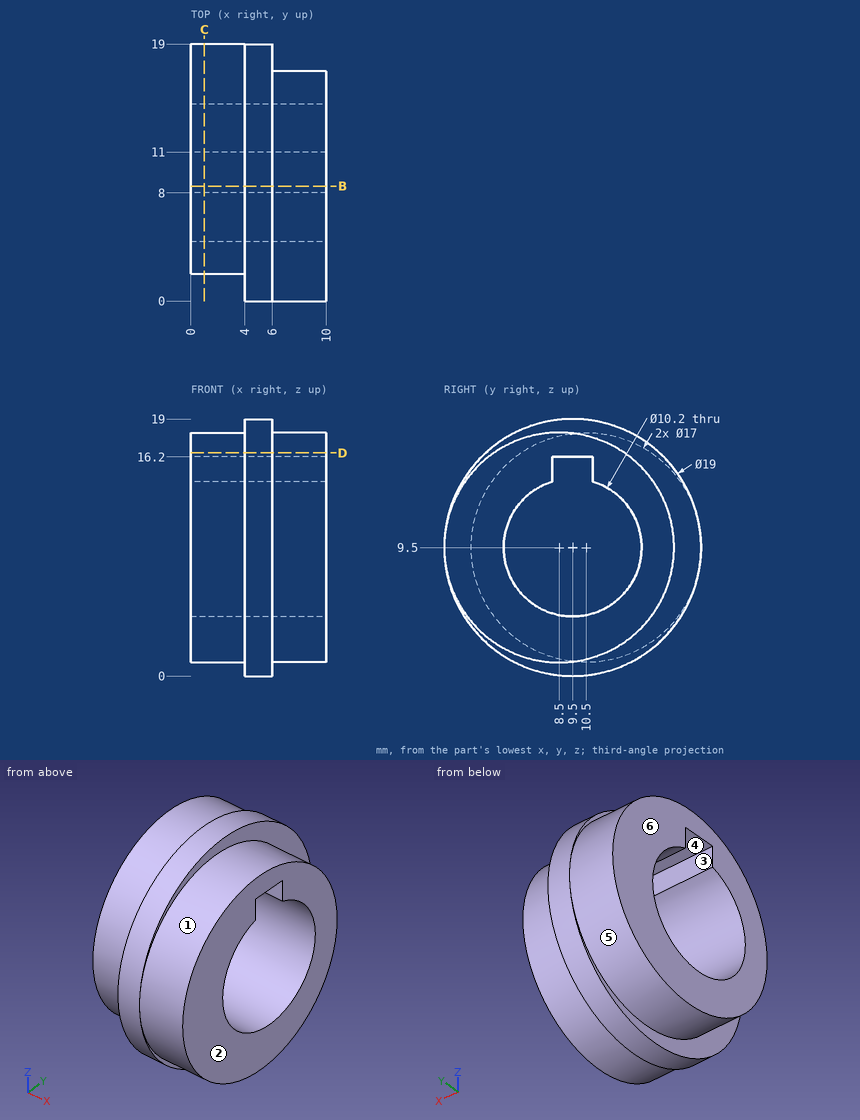
Geometry check sheet. Reference: drawing and pictorial views, mm from the part's lowest x, y, z. A direction names the side the tool comes from. Give positions to 0.01 mm unless a question says otherwise; leave off trailing zeros. Order: outer loops, then holes, each group sorted by start corner. A loop starts at its lowest first (then second) coordinate and runs counter-clockwise, first axis right, second up. Notation, with made-up numbers: M -4.5,69 L 21.5,69 A31 cw 21.5,108 Z; hole C -3,-32.75 d9. An arc over 180 degrees is marked long. Answer in a Markdown table with one row per item. Add a question column.
Q1. Sectioned sample at B-B, the plane y = 8.5. Record the boundary of the cut face in (x, z).
Q2. Access from +Z, -Z, +X, -X, +Y, -Y to the whole of each face (thin tool, end or side, straight path). Record for the marked faces 4, 5 and 6.
Q3. Sectioned sample at D-D, the plane z = 16.5. Record the boundary of the cut face in (x, y), and give its area (3 significant figures).
Q4. Thickness scan on L1, parallel to Z at x = 5, y = 9.5; L2, parallel to Y at x = 3.25, z = 9.5; L3, parallel to Z at x = 7.75, y = 7.25. Record the ranges inside material, lowest first.
Q5. Gauge pin test, flat ends, axial feed: pin 1 Ø1.5 at (x, y) = (8.5, 10) entering from -Z; pin 2 Ø6 at (y, z) = (16.5, 16.5) entering from -X; pin 3 Ø0.9 at (x, z) = (4, 15.5) entering from +Y; pin 4 Ø4 at (x, z) = (3, 17) entering from -Y. Record the tip position at first contact, or that the pin passes through.
Q6. Release check for a two-part mould opening along Z. For the marked faces 1, 2 and 3 record: released by +Z, released by -Z, zero draft, split by the parting line, or undercut.
Q7. Sectioned sample at C-C, the plane x = 1. Record the boundary of the cut face in (y, z), and give its area (3 significant figures).
Verdict:
| question | item | result |
|---|---|---|
| 1 | outline | M 0,1.24 L 4,1.24 L 4,0.05 L 6,0.05 L 6,1 L 10,1 L 10,4.5 L 0,4.5 Z; M 0,16.2 L 10,16.2 L 10,18 L 6,18 L 6,18.95 L 4,18.95 L 4,17.76 L 0,17.76 Z |
| 2 | face 4 | +X, -X |
| 2 | face 5 | -X |
| 2 | face 6 | +Z, -Z, -X, +Y, -Y |
| 3 | outline | M 0,5.68 L 4,5.68 L 4,3.08 L 6,3.08 L 6,3.68 L 10,3.68 L 10,13.32 L 6,13.32 L 6,15.92 L 4,15.92 L 4,15.32 L 0,15.32 Z |
| 3 | area | 103 mm² |
| 4 | L1 | 0 to 4.4, 16.2 to 19 |
| 4 | L2 | 2 to 4.4, 14.6 to 19 |
| 4 | L3 | 1.09 to 4.92, 14.08 to 17.91 |
| 5 | pin 1 | z = 1.03 |
| 5 | pin 2 | x = 0 |
| 5 | pin 3 | y = 17.21 |
| 5 | pin 4 | y = 1.95 |
| 6 | face 1 | split by the parting line |
| 6 | face 2 | zero draft |
| 6 | face 3 | undercut |
| 7 | outline | C 10.5,9.5 d17; hole M 8,14.37 A5.1 ccw long 11,14.37 L 11,16.2 L 8,16.2 Z |
| 7 | area | 140 mm² |
